Source: CAD feature listing. Evaluate the final solid. Frame: model axes, mm. Round coordinates to 2 decimals unless told otherwise and drop trailing zeros. Loops run counter-clockwise (first coordinate to the right, second up) from the corner with the lowest first, then second, coordinate; pieces in that order, holes last. Notation, with made-up numbers: (2, -38) - (14, -38) arc R5 cw to (14, -34) - close; hole circle Ø4 at (65.5, -8.5). An arc over 180 degrees is marked (long way). One line per question, with ' | ' between items.
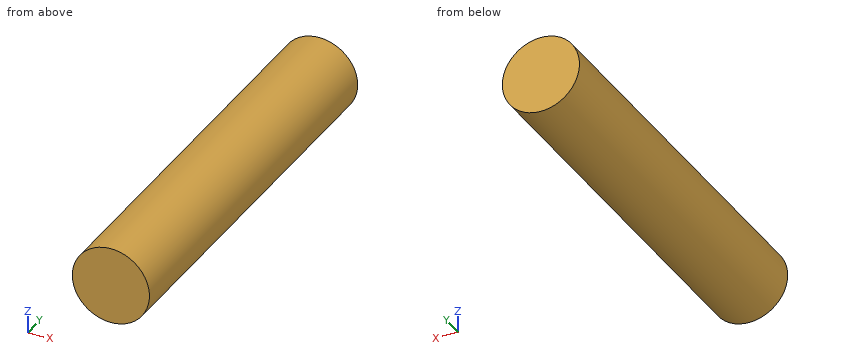
Autodesk Inventor part; units mm, degrees
ref_plane "YZ Plane" through (0, 0, 0) normal (1, 0, 0) x (0, 1, 0)
ref_plane "XZ Plane" through (0, 0, 0) normal (0, 1, 0) x (-1, 0, 0)
ref_plane "XY Plane" through (0, 0, 0) normal (0, 0, 1) x (1, 0, 0)
sketch "スケッチ1" plane through (0, 0, 0) normal (0, 1, 0) x (-1, 0, 0)
  circle A0 centre (0, 0) radius 7
  dimension "d0" = 14
extrude "押し出し1" add sketch "スケッチ1" along normal blind 70
sketch "スケッチ2" plane through (0, 70, 0) normal (0, 1, 0) x (1, 0, 0)
  circle A0 centre (0, 0) radius 7
sketch "スケッチ3" plane through (0, 70, 0) normal (0, 1, 0) x (1, 0, 0)
  circle A0 centre (0, 0) radius 7
  circle A1 centre (0, 0) radius 27.5
  dimension "d3" = 55
extrude "押し出し2" add sketch "スケッチ3" along normal blind 3
extrude "押し出し3" add sketch "スケッチ2" along normal blind 3
sketch "スケッチ4" plane through (0, 73, 0) normal (0, 1, 0) x (1, 0, 0)
  circle A0 centre (0, 0) radius 27.5
  circle A1 centre (0, 0) radius 25
  line L0 (0, 0) -> (17.6777, 17.6777)
  line L1 (0, 0) -> (25, 0) construction
  circle A2 centre (17.6777, 17.6777) radius 1.5
  circle A3 centre (-17.6777, 17.6777) radius 1.5
  circle A4 centre (-17.6777, -17.6777) radius 1.5
  circle A5 centre (17.6777, -17.6777) radius 1.5
  dimension "d8" = 50
  dimension "d9" = 45
  dimension "d10" = 3
  dimension "d13" = 360
hole "穴1" at (0, 73, 0) at (-17.6777, 73, -17.6777) at (17.6777, 73, -17.6777) at (17.6777, 73, 17.6777) at (-17.6777, 73, 17.6777) direction (0, -1, 0) diameter 3 depth 8 tip angle 118
sketch "スケッチ6" plane through (0, 70, 0) normal (0, -1, 0) x (1, 0, 0)
  circle A0 centre (17.6777, 17.6777) radius 1.5
  circle A1 centre (-17.6777, -17.6777) radius 1.5
  circle A2 centre (17.6777, -17.6777) radius 1.5
  circle A3 centre (-17.6777, 17.6777) radius 1.5
  circle A4 centre (0, 0) radius 7
  circle A5 centre (0, 0) radius 27.5
extrude "押し出し5" cut sketch "スケッチ6" against normal blind 3
sketch "スケッチ7" plane through (0, 73, 0) normal (0, 1, 0) x (1, 0, 0)
  circle A0 centre (0, 0) radius 1.5
  circle A1 centre (0, 0) radius 1.5
extrude "押し出し6" add sketch "スケッチ7" against normal blind 73
properties part number "知能ロボコンばね受け"
1. Contact query for flat-ended pins moving along their axis: P1, Ø1.5, axis at y = 61, z = 4, coming from the +X side; P2, Ø2, axis at y = 32.5, z = 3.5, coming from the -X side; P3, Ø4, axis at x = 3.5, y = 34, coming from the +Z side. Output: stop coordinate, or through.
Worked out:
P1: stops at x = 6.2 | P2: stops at x = -6.54 | P3: stops at z = 6.84
2. Material intervals for probe 1 along Z at (x, y) = (-0.25, 66); probe 2 along Z at (x, y) = (3, 38.5); probe 3 along X at (y, z) = (30, 3.25), sorted ascending.
Worked out:
probe 1: z = -7 to 7 | probe 2: z = -6.32 to 6.32 | probe 3: x = -6.2 to 6.2
3. Section query B-B, the plane x = 5.5. Return loops of the section in (y, z), plus the area to 3 significant figures.
Worked out:
outline: (0, -4.33) - (73, -4.33) - (73, 4.33) - (0, 4.33) - close | area: 632 mm2
4. Section query C-C, the plane z = 4. Return loops of the section in (x, y), plus the area to 3 significant figures.
Worked out:
outline: (-5.74, 0) - (5.74, 0) - (5.74, 73) - (-5.74, 73) - close | area: 839 mm2
5. Section query A-A, the plane y = 32. Return loops of the section in (x, z).
Worked out:
outline: circle Ø14 at (0, 0)
